```python
from build123d import *

# Parameters (mm, degrees)
SKETCH1_W           = 15.1
SKETCH1_H           = 20
BOSS_EXTRUDE1_DEPTH = 7.7
BOSS_EXTRUDE2_DEPTH = 1.5
SKETCH4_R           = 1.5
CUT_EXTRUDE1_DEPTH  = 18.984785236


with BuildPart() as part:
    # Sketch1 → Boss-Extrude1 (new body)
    with BuildSketch(Plane.XY):
        Rectangle(SKETCH1_W, SKETCH1_H)
    extrude(amount=BOSS_EXTRUDE1_DEPTH)

    # Sketch3 → Boss-Extrude2 (add)
    with BuildSketch(Plane(origin=(0, 0, 0), x_dir=(-1, 0, 0), z_dir=(0, 0, -1))):
        Polygon((4.605513627, 15.1), (-4.605513627, 15.1), (-7.55, 10), (7.55, 10), align=None)
    extrude(amount=-BOSS_EXTRUDE2_DEPTH)

    # Sketch4 → Cut-Extrude1 (cut, through all)
    with BuildSketch(Plane.XY.offset(1.5)):
        with Locations((0, 11.9)):
            Circle(SKETCH4_R)
    extrude(amount=-CUT_EXTRUDE1_DEPTH, mode=Mode.SUBTRACT)


solid = part.part
```
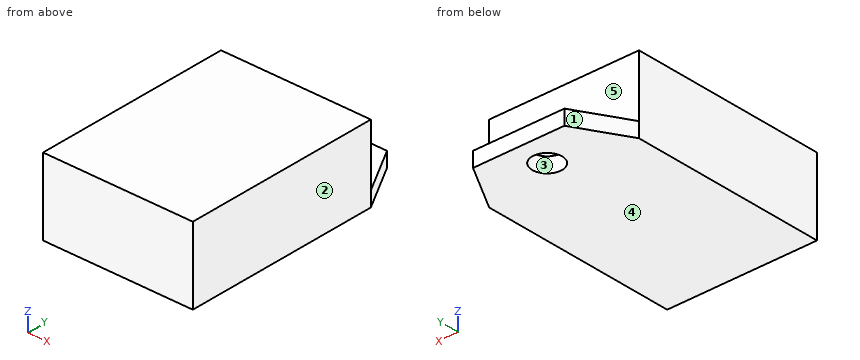
The model under review builds one solid part; all positions refer to its coordinate system, in mm. Face numbers are marked on the shaded views. A direction names the side the tool comes from. Give positions to 0.01 mm unless a question says otherwise; leave off trailing zeros. Order: outer loops, then holes, each group sorted by start corner. A loop starts at its lowest first (then second) coordinate and runs counter-clockwise, first axis right, second up. Notation, with made-up numbers: (53.5, -16.5) - (62.5, -16.5) arc R20 cw to (62.5, 21.5) - close; hole circle Ø2 at (-17, -32). An arc over 180 degrees is marked (long way). Use CSV: the item, a comma, the result in double quotes. Start each with the question number.
Q1. We need section D-D, the plane z = 5.5. Write out the cut boundary in (x, y), and give its area (3 significant figures).
Q2. We need section C-C, the plane y = 11.9. Write out the cut boundary in (x, z), and give its area (3 significant figures).
Q3. To check wall thickness, follow line 1 along Y through (x, z) = (0, 0.7); line 2 along Y through (x, z) = (0.25, 6.5); line 3 along Z through (x, y) = (-1.75, 10.5). State the ranges of each line that lie inside material, in increasing order. Write a range as [from, to].
Q4. Clearance check with flat-ended pins moving along their axes: pin 1 Ø3 at (x, z) = (-2, 4) entering from +Y; pin 2 Ø1.8 at (x, y) = (0, 11.9) entering from -Z. State where each tip first meets the part, or that it passes through.
Q5. We need section B-B, the plane x = 0. Write out the cut boundary in (y, z), and give its area (3 significant figures).
Q6. The part is to be moulded in two halves that separate along X. For the marked faces 1, 2 and 3, say which applies: +X half, -X half, draft (parallel to the pull), parting line (faces both ways), or undercut.
Q7. Tool access review of the marked faces 4 and 5: name each direction out of +Z, -Z, +X, -X, +Y, -Y from which nothing blocks a thin tool from reaching the whole face with its end or side.
Q8. We need section A-A, the plane z = 0.5. Write out the cut boundary in (x, y), and give its area (3 significant figures).
Outcome:
1,outline,"(-7.55, -10) - (7.55, -10) - (7.55, 10) - (-7.55, 10) - close"
1,area,"302 mm^2"
2,outline,"(-6.45, 0) - (-1.5, 0) - (-1.5, 1.5) - (-6.45, 1.5) - close; (1.5, 0) - (6.45, 0) - (6.45, 1.5) - (1.5, 1.5) - close"
2,area,"14.9 mm^2"
3,line 1,"y = [-10, 10.4], [13.4, 15.1]"
3,line 2,"y = [-10, 10]"
3,line 3,"z = [0, 1.5]"
4,pin 1,"stops at y = 10"
4,pin 2,"passes through"
5,outline,"(-10, 0) - (10.4, 0) - (10.4, 1.5) - (10, 1.5) - (10, 7.7) - (-10, 7.7) - close; (13.4, 0) - (15.1, 0) - (15.1, 1.5) - (13.4, 1.5) - close"
5,area,"157 mm^2"
6,face 1,"-X half"
6,face 2,"+X half"
6,face 3,"undercut"
7,face 4,"-Z, +X, -X, +Y, -Y"
7,face 5,"+Z, +X, -X, +Y"
8,outline,"(-7.55, -10) - (7.55, -10) - (7.55, 10) - (4.61, 15.1) - (-4.61, 15.1) - (-7.55, 10) - close; hole circle Ø3 at (0, 11.9)"
8,area,"357 mm^2"
